Here's how the part is built. I have some questions about the finished solid (model axes, mm). A direction names the side the tool comes from. Coordinates: 2 decimals unless noted, no trailing zeros. Order: outer loops, then holes, each group sorted by start corner. A loop starts at its lowest first (then second) coordinate and runs counter-clockwise, first axis right, second up. Notation, with made-up numbers: (-28.75, 6) - (18.25, 6) arc R22 ccw to (18.25, 30) - close; hole circle Ø5 at (-30.75, 33). An arc over 180 degrees is marked (long way). Use CSV: the item, a comma, the result in double quotes. Start each with the question number.
from build123d import *

# Parameters (mm, degrees)
SKETCH_1_W              = 36
SKETCH_1_H              = 18
EXTRUDE_1_DEPTH         = 8
CUT_EXTRUDE_1_DEPTH     = 38.960505792
CHAMFER_1_SIZE          = 2
CUT_EXTRUDE_2_DEPTH     = 22.656407828
CUT_EXTRUDE_START       = -2
CUT_EXTRUDE_3_OUTLINE_R = 2
CUT_EXTRUDE_3_DEPTH     = 2
EXTRUDE_2_DEPTH         = 0.2
EXTRUDE_3_DEPTH         = 3
SKETCH_7_W              = 6
SKETCH_7_H              = 6.2
CUT_EXTRUDE_4_DEPTH     = 0.5
CHAMFER_16_SIZE         = 0.5
CUT_EXTRUDE_5_REACH     = 28.683


# Read off the part's stored shape, not the designer's step: Вырез-Вытянуть3
with BuildPart() as part:
    # Эскиз1 → Бобышка-Вытянуть1 (new body)
    with BuildSketch(Plane(origin=(0, 0, 0), x_dir=(0, 0, -1), z_dir=(1, 0, 0))):
        Rectangle(SKETCH_1_W, SKETCH_1_H)
    extrude(amount=EXTRUDE_1_DEPTH)

    # Эскиз2 → Вырез-Вытянуть1 (cut, through all)
    with BuildSketch(Plane.XY.offset(18)):
        with BuildLine():
            ThreePointArc((0, -3.1), (3.1, 0), (0, 3.1))
            Line((0, 3.1), (0, -3.1))
        make_face()
    extrude(amount=-CUT_EXTRUDE_1_DEPTH, mode=Mode.SUBTRACT)

    # Фаска1
    chamfer_1_edges = [part.edges().sort_by_distance(p)[0] for p in [
        (8, 0, 18),
        (8, -9, 0),
        (8, 0, -18),
        (8, 9, 0),
    ]]
    chamfer(chamfer_1_edges, length=CHAMFER_1_SIZE)

    # Эскиз3 → Вырез-Вытянуть2 (cut, through all)
    with BuildSketch(Plane(origin=(8, 0, 0), x_dir=(0, 0, -1), z_dir=(1, 0, 0))):
        with BuildLine():
            ThreePointArc((1.413329403, 7), (1.552631161, 6.636440782), (1.6, 6.25))
            ThreePointArc((1.6, 6.25), (-0.386440782, 4.697368839), (-1.413329403, 7))
            Line((-1.413329403, 7), (-1.854049622, 7))
            ThreePointArc((-1.854049622, 7), (-0.382034525, 4.286826645), (2, 6.25))
            ThreePointArc((2, 6.25), (1.963173355, 6.632034525), (1.854049622, 7))
            Line((1.854049622, 7), (1.413329403, 7))
        make_face()
        with BuildLine():
            ThreePointArc((-1.413329403, 7), (0, 7.85), (1.413329403, 7))
            Line((1.413329403, 7), (1.854049622, 7))
            ThreePointArc((1.854049622, 7), (0, 8.25), (-1.854049622, 7))
            Line((-1.854049622, 7), (-1.413329403, 7))
        make_face()
        with BuildLine():
            ThreePointArc((-1.413329403, 7), (-0.386440782, 4.697368839), (1.6, 6.25))
            ThreePointArc((1.6, 6.25), (1.552631161, 6.636440782), (1.413329403, 7))
            Line((1.413329403, 7), (-1.413329403, 7))
        make_face()
        with BuildLine():
            Line((-1.413329403, 7), (1.413329403, 7))
            ThreePointArc((1.413329403, 7), (0, 7.85), (-1.413329403, 7))
        make_face()
        with BuildLine():
            ThreePointArc((-1.413329403, -7), (-0.386440782, -4.697368839), (1.6, -6.25))
            ThreePointArc((1.6, -6.25), (1.552631161, -6.636440782), (1.413329403, -7))
            Line((1.413329403, -7), (1.854049622, -7))
            ThreePointArc((1.854049622, -7), (1.963173355, -6.632034525), (2, -6.25))
            ThreePointArc((2, -6.25), (-0.382034525, -4.286826645), (-1.854049622, -7))
            Line((-1.854049622, -7), (-1.413329403, -7))
        make_face()
        with BuildLine():
            ThreePointArc((1.413329403, -7), (0, -7.85), (-1.413329403, -7))
            Line((-1.413329403, -7), (-1.854049622, -7))
            ThreePointArc((-1.854049622, -7), (0, -8.25), (1.854049622, -7))
            Line((1.854049622, -7), (1.413329403, -7))
        make_face()
        with BuildLine():
            ThreePointArc((1.413329403, -7), (1.552631161, -6.636440782), (1.6, -6.25))
            ThreePointArc((1.6, -6.25), (-0.386440782, -4.697368839), (-1.413329403, -7))
            Line((-1.413329403, -7), (1.413329403, -7))
        make_face()
        with BuildLine():
            Line((1.413329403, -7), (-1.413329403, -7))
            ThreePointArc((-1.413329403, -7), (0, -7.85), (1.413329403, -7))
        make_face()
    extrude(amount=-CUT_EXTRUDE_2_DEPTH, mode=Mode.SUBTRACT)

    # Вырез-Вытянуть3 outline → Вырез-Вытянуть3 (cut)
    # profile 1 of 2: a face of its own
    with BuildSketch(Plane(origin=(8, 0, 0), x_dir=(0, 0, -1), z_dir=(1, 0, 0)).offset(CUT_EXTRUDE_START)):
        with BuildLine():
            Line((-3, 9), (-3, 6.25))
            ThreePointArc((-3, 6.25), (0, 3.25), (3, 6.25))
            Line((3, 6.25), (3, 9))
            Line((3, 9), (-3, 9))
        make_face()
        with Locations((0, 6.25)):
            Circle(CUT_EXTRUDE_3_OUTLINE_R, mode=Mode.SUBTRACT)
    # profile 2 of 2: a face of its own
    with BuildSketch(Plane(origin=(8, 0, 0), x_dir=(0, 0, -1), z_dir=(1, 0, 0)).offset(CUT_EXTRUDE_START)):
        with BuildLine():
            Line((3, -9), (3, -6.25))
            ThreePointArc((3, -6.25), (0, -3.25), (-3, -6.25))
            Line((-3, -6.25), (-3, -9))
            Line((-3, -9), (3, -9))
        make_face()
        with Locations((0, -6.25)):
            Circle(CUT_EXTRUDE_3_OUTLINE_R, mode=Mode.SUBTRACT)
    extrude(amount=CUT_EXTRUDE_3_DEPTH, mode=Mode.SUBTRACT)

    # Эскиз5 → Бобышка-Вытянуть2 (add)
    with BuildSketch(Plane(origin=(6, 0, 0), x_dir=(0, 0, -1), z_dir=(1, 0, 0))):
        with BuildLine():
            Line((3, 9), (-3, 9))
            Line((-3, 9), (-3, 6.25))
            ThreePointArc((-3, 6.25), (0, 3.25), (3, 6.25))
            Line((3, 6.25), (3, 9))
        make_face()
        with BuildLine():
            Line((-3, -9), (3, -9))
            Line((3, -9), (3, -6.25))
            ThreePointArc((3, -6.25), (0, -3.25), (-3, -6.25))
            Line((-3, -6.25), (-3, -9))
        make_face()
    extrude(amount=EXTRUDE_2_DEPTH)

    # Эскиз6 → Бобышка-Вытянуть3 (add, symmetric)
    with BuildSketch(Plane.XY):
        with BuildLine():
            Line((0, 3.1), (0, -3.1))
            ThreePointArc((0, -3.1), (3.1, 0), (0, 3.1))
        make_face()
    extrude(amount=EXTRUDE_3_DEPTH, both=True)

    # Эскиз7 → Вырез-Вытянуть4 (cut, symmetric)
    with BuildSketch(Plane.ZY):
        Rectangle(SKETCH_7_W, SKETCH_7_H)
    extrude(amount=CUT_EXTRUDE_4_DEPTH, both=True, mode=Mode.SUBTRACT)

    # Фаска16
    # the kernel refuses this chamfer: 0.5 mm, written as the material it adds along each edge
    with BuildSketch(Plane(origin=(0.5, 3.1, 3), x_dir=(-0.9996219169112968, 0.027495876610586494, 0), z_dir=(0, 0, -1))) as chamfer_16_piece_1_section:
        Polygon((CHAMFER_16_SIZE * 0.999621916911, -CHAMFER_16_SIZE * 0.0274958766106), (-CHAMFER_16_SIZE * 0.0274958766106, -CHAMFER_16_SIZE * 0.999621916911), (0, 0), align=None)
    chamfer_16_piece_1 = extrude(amount=6, mode=Mode.PRIVATE)
    chamfer_16_piece_1 = split(chamfer_16_piece_1, bisect_by=Plane(origin=(0, 2.934797923, 0), z_dir=(1, 0, 0)), keep=Keep.TOP, mode=Mode.PRIVATE)
    add(chamfer_16_piece_1)
    with BuildSketch(Plane(origin=(0.5, -3.1, -3), x_dir=(-0.9996219169112968, -0.027495876610586494, 0), z_dir=(0, 0, 1))) as chamfer_16_piece_2_section:
        Polygon((CHAMFER_16_SIZE * 0.999621916911, -CHAMFER_16_SIZE * 0.0274958766106), (-CHAMFER_16_SIZE * 0.0274958766106, -CHAMFER_16_SIZE * 0.999621916911), (0, 0), align=None)
    chamfer_16_piece_2 = extrude(amount=6, mode=Mode.PRIVATE)
    chamfer_16_piece_2 = split(chamfer_16_piece_2, bisect_by=Plane(origin=(0, -2.934797923, 0), z_dir=(1, 0, 0)), keep=Keep.TOP, mode=Mode.PRIVATE)
    add(chamfer_16_piece_2)

    # Вырез-Вытянуть5: up to this plane
    cut_extrude_5_end = Plane(origin=(0.5, -2.6, 0), z_dir=(0.7071067811865525, -0.7071067811865426, 0))
    # Эскиз8 → Вырез-Вытянуть5 (cut, up to the surface)
    with BuildSketch(Plane.XZ.offset(9), mode=Mode.PRIVATE) as cut_extrude_5_sk1:
        with BuildLine():
            ThreePointArc((3.5, 6.75), (2.474873734, 9.224873734), (0, 10.25))
            Line((0, 10.25), (0, 3.25))
            ThreePointArc((0, 3.25), (2.474873734, 4.275126266), (3.5, 6.75))
        make_face()
    cut_extrude_5_tool1 = split(extrude(cut_extrude_5_sk1.sketch, amount=-CUT_EXTRUDE_5_REACH, mode=Mode.PRIVATE), bisect_by=cut_extrude_5_end, keep=Keep.BOTH, mode=Mode.PRIVATE)
    add(cut_extrude_5_tool1.solids().sort_by_distance((1.485446, -9, 6.75))[0], mode=Mode.SUBTRACT)
    # Эскиз8 → Вырез-Вытянуть5 (cut, up to the surface)
    with BuildSketch(Plane.XZ.offset(9), mode=Mode.PRIVATE) as cut_extrude_5_sk2:
        with BuildLine():
            Line((0, 3.25), (0, 10.25))
            ThreePointArc((0, 10.25), (-3.5, 6.75), (0, 3.25))
        make_face()
    cut_extrude_5_tool2 = split(extrude(cut_extrude_5_sk2.sketch, amount=-CUT_EXTRUDE_5_REACH, mode=Mode.PRIVATE), bisect_by=cut_extrude_5_end, keep=Keep.BOTH, mode=Mode.PRIVATE)
    add(cut_extrude_5_tool2.solids().sort_by_distance((-1.485446, -9, 6.75))[0], mode=Mode.SUBTRACT)
    # Эскиз8 → Вырез-Вытянуть5 (cut, up to the surface)
    with BuildSketch(Plane.XZ.offset(9), mode=Mode.PRIVATE) as cut_extrude_5_sk3:
        with BuildLine():
            ThreePointArc((3.5, -6.75), (2.474873734, -4.275126266), (0, -3.25))
            Line((0, -3.25), (0, -10.25))
            ThreePointArc((0, -10.25), (2.474873734, -9.224873734), (3.5, -6.75))
        make_face()
    cut_extrude_5_tool3 = split(extrude(cut_extrude_5_sk3.sketch, amount=-CUT_EXTRUDE_5_REACH, mode=Mode.PRIVATE), bisect_by=cut_extrude_5_end, keep=Keep.BOTH, mode=Mode.PRIVATE)
    add(cut_extrude_5_tool3.solids().sort_by_distance((1.485446, -9, -6.75))[0], mode=Mode.SUBTRACT)
    # Эскиз8 → Вырез-Вытянуть5 (cut, up to the surface)
    with BuildSketch(Plane.XZ.offset(9), mode=Mode.PRIVATE) as cut_extrude_5_sk4:
        with BuildLine():
            Line((0, -10.25), (0, -3.25))
            ThreePointArc((0, -3.25), (-3.5, -6.75), (0, -10.25))
        make_face()
    cut_extrude_5_tool4 = split(extrude(cut_extrude_5_sk4.sketch, amount=-CUT_EXTRUDE_5_REACH, mode=Mode.PRIVATE), bisect_by=cut_extrude_5_end, keep=Keep.BOTH, mode=Mode.PRIVATE)
    add(cut_extrude_5_tool4.solids().sort_by_distance((-1.485446, -9, -6.75))[0], mode=Mode.SUBTRACT)


solid = part.part
Item 1: Suppose I cut it at C-C on z = 0. Write out the boundary of the cut face in (x, y).
Item 2: Suppose I cut it at D-D on x = 6.75. Write out the boundary of the cut face in (y, z).
Item 3: For pin 1 Ø1.4 at (x, y) = (7.5, -8) entering from -Z; pin 2 Ø3.5 at (y, z) = (-6.25, 0) entering from -X; pin 3 Ø1.7 at (y, z) = (7.5, -0.5) entering from +X, each with a flat end and sliding along its axis, tell me the tip position at first contact or that it passes through.
Item 4: Please list where these lines run through material, in increasing order: line 1 along Z through (x, y) = (2, 6.25); line 2 along X through (y, z) = (8, 4.5); line 3 along Y through (x, z) = (6.75, -7). Write a range as from..to.
Item 5: Suppose I cut it at A-A on x = 2.25. Write out the boundary of the cut face in (y, z), then the cut area to 3 significant figures.
Item 6: Suppose I cut it at B-B on x = 4.25. Write out the boundary of the cut face in (y, z), then the cut area to 3 significant figures.
Item 7: We'd pull the mould along Y, two halves only. Please class faces 5 (the flat face through (0, 4, 0)), 6 (the flat face through (7, -8, -10)), 7 (the flat face through (1, 0, -3)), 8 (the cylindrical face through (7.09, 3.25, 0.07)): released by +Y, released by -Y, zero draft, split by the parting line, or undercut.
Item 8: For faces 1 (the cylindrical face through (2.936, 0.996, -12.062)), 2 (the flat face through (6, 6, 0)), 3 (the flat face through (1, 0, 3)), 4 (the flat face through (7, -7, -3)), which set-ups out of +Z, -Z, +X, -X, +Y, -Y let a thin tool reach every point of the face, with its end or its side?
Here are the results:
1,outline,"(0, -9) - (6.2, -9) - (6.2, -3.25) - (8, -3.25) - (8, 3.25) - (6.2, 3.25) - (6.2, 9) - (0, 9) - (0, 8.25) - (6, 8.25) - (6, 4.25) - (0, 4.25) - (0, 3.1) - (0.5, 2.6) - (0.5, -2.6) - (0, -3.1) - (0, -4.25) - (6, -4.25) - (6, -8.25) - (0, -8.25) - close"
2,outline,"(-8.25, -17.25) - (8.25, -17.25) - (8.25, -3) - (6.25, -3) arc R3 cw to (6.25, 3) - (8.25, 3) - (8.25, 17.25) - (-8.25, 17.25) - (-8.25, 3) - (-6.25, 3) arc R3 cw to (-6.25, -3) - (-8.25, -3) - close"
3,pin 1,"z = -17.2"
3,pin 2,"x = 6"
3,pin 3,"x = 6.2"
4,line 1,"-18..-2, 2..18"
4,line 2,"0..7"
4,line 3,"-8.25..8.25"
5,outline,"(-9, -18) - (-2.13, -18) - (-2.13, -9.43) - (-9, -9.43) - close; (-9, -4.07) - (-2.13, -4.07) - (-2.13, -3) - (2.13, -3) - (2.13, -18) - (9, -18) - (9, 18) - (2.13, 18) - (2.13, 3) - (-2.13, 3) - (-2.13, 4.07) - (-9, 4.07) - close; (-9, 9.43) - (-2.13, 9.43) - (-2.13, 18) - (-9, 18) - close; hole circle Ø4 at (-6.25, 0); hole circle Ø4 at (6.25, 0)"
5,area,"421 mm^2"
6,outline,"(-9, -18) - (9, -18) - (9, 18) - (-9, 18) - close; hole circle Ø4 at (-6.25, 0); hole circle Ø4 at (6.25, 0)"
6,area,"623 mm^2"
7,face 5,"zero draft"
7,face 6,"released by -Y"
7,face 7,"undercut"
7,face 8,"released by +Y"
8,face 1,"-Z, -X"
8,face 2,"-X"
8,face 3,"+Z, -X"
8,face 4,"+X, -Y"
